Job drawing, mm, ordinate dimensions from the low corner. One solid piece. A direction names the side the tool comes from. Give positions to 0.01 mm unless a question says otherwise; leave off trailing zeros. Order: outer loops, then holes, each group sorted by start corner. A loop starts at its lowest first (then second) coordinate and runs counter-clockwise, first axis right, second up. Notation, with made-up numbers: M 57.25,67 L 69.25,67 A25 ccw 69.25,80 Z; hole C -23.75,4.5 d6. An arc over 180 degrees is marked long. One line per question, with ' | ' between items.
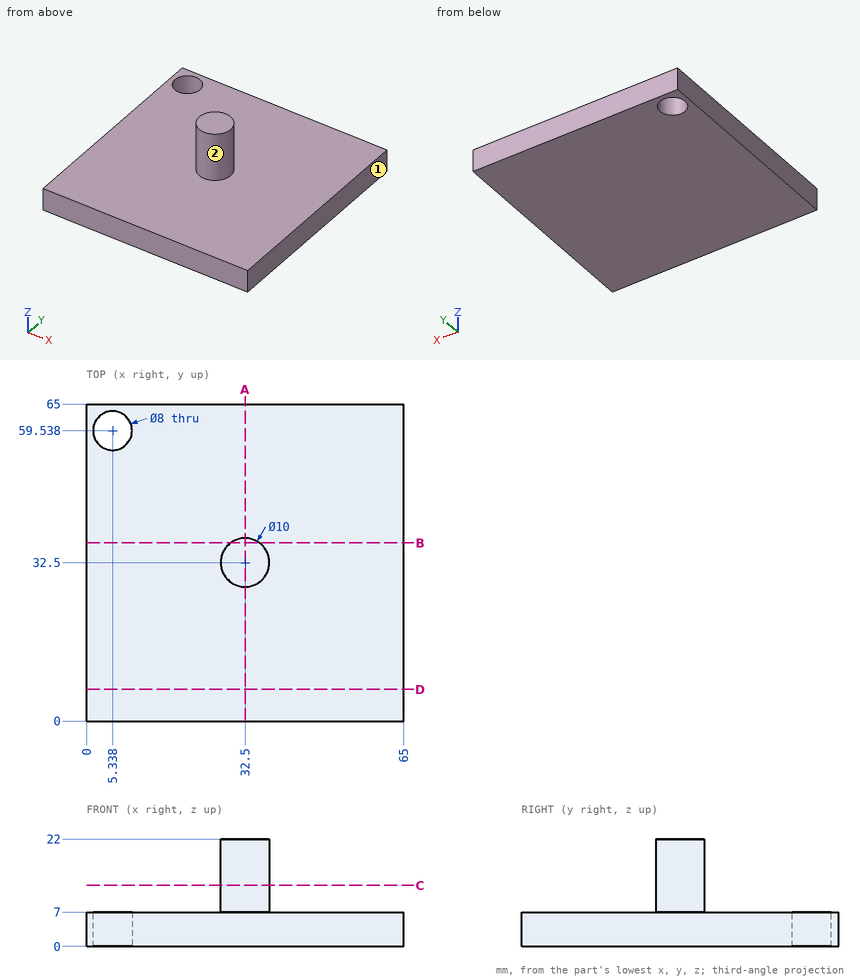
1. Probe L1, parallel to Z at x = 9, y = 27.5; L2, parallel to Y at x = 6, z = 5.5; L3, parallel to X at y = 61, z = 3.25 (1 decimal). List the from-to ranges inside material, lowest first. Write a range as from..to.
Worked out:
L1: z = 0..7 | L2: y = 0..55.59, 63.48..65 | L3: x = 0..1.6, 9.1..65
2. Slice it at A-A on x = 32.5. Give the cut face in (y, z), then the cut area to 3 significant figures.
Worked out:
outline: M 0,0 L 65,0 L 65,7 L 37.5,7 L 37.5,22 L 27.5,22 L 27.5,7 L 0,7 Z | area: 605 mm2
3. Drop flat-ended pins along their axis: pin 1 (3 mm diameter, centred on x = 34.5, y = 41.5, fed in from +Z); pin 2 (5 mm diameter, centred on y = 8, z = 10.5, fed in from +X). Give the stop position or say it passes through.
Worked out:
pin 1: stops at z = 7 | pin 2: passes through
4. Slice it at D-D on y = 6.5. Give the cut face in (x, z).
Worked out:
outline: M 0,0 L 65,0 L 65,7 L 0,7 Z
5. Tool access for the marked faces 1 and 2: list every direction of +Z, -Z, +X, -X, +Y, -Y with a clear straight run to the whole face (end or side of a thin tool).
Worked out:
face 1: +Z, -Z, +X, +Y, -Y | face 2: +Z
6. Slice it at B-B on y = 36.5. Give the cut face in (x, z).
Worked out:
outline: M 0,0 L 65,0 L 65,7 L 35.5,7 L 35.5,22 L 29.5,22 L 29.5,7 L 0,7 Z
7. Slice it at C-C on z = 12.5. Give the cut face in (x, y).
Worked out:
outline: C 32.5,32.5 d10
